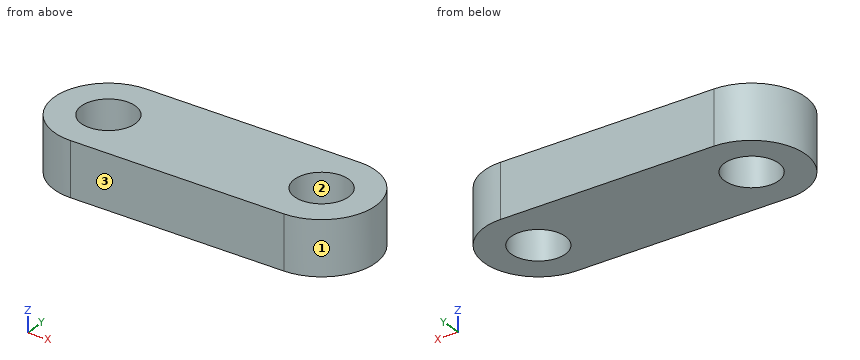
```python
from build123d import *

# Parameters (mm, degrees)
BASE_EXTRUDE_DEPTH              = 3.175
F_1_4_0_250000_DIAMETER_HOLE1_D = 6.35


with BuildPart() as part:
    # profile → Base-Extrude (new body, symmetric)
    with BuildSketch(Plane.XY):
        with BuildLine():
            Line((-25.4, 6.35), (0, 6.35))
            ThreePointArc((0, 6.35), (6.35, 0), (0, -6.35))
            Line((0, -6.35), (-25.4, -6.35))
            ThreePointArc((-25.4, -6.35), (-31.75, 0), (-25.4, 6.35))
        make_face()
    extrude(amount=BASE_EXTRUDE_DEPTH, both=True)

    # 1/4 (0.250000) Diameter Hole1 (through all)
    with Locations(Plane.XY.offset(3.175)):
        with Locations((-25.4, 0), (0, 0)):
            Hole(F_1_4_0_250000_DIAMETER_HOLE1_D / 2)


solid = part.part
```
Check sheet for the modelled part. Datum: model origin and axes. Units: mm. Face numbers are marked on the shaded views. Coordinates: 2 decimals unless noted, no trailing zeros. Order: outer loops, then holes, each group sorted by start corner. A loop starts at its lowest first (then second) coordinate and runs counter-clockwise, first axis right, second up. Notation, with made-up numbers: (-17, 60) -> (40, 60) arc R7 ccw to (40, 71) -> close; hole circle Ø5 at (48.5, 65.5). An arc over 180 degrees is marked (long way). Write item = value, one per line. Start each with the question number.
1) Cross-section at B-B (z = -1.25). Enter the section's corners in (x, y) (3 decimals).
2) Go/stop test with a flat-tipped pin: P1, Ø1.5, axis at y = -4, z = 0.5, coming from the +X side. Record where the tip stops, or that it passes through.
3) Cross-section at D-D (y = -2.25). Enter the section's corners in (x, z) (3 decimals).
4) Mould release check, pull along Y, two halves, no side actions. Record for the marked faces 1, 2 and 3: +Y half, -Y half, draft (parallel to the pull), parting line (faces both ways), or undercut.
5) Material ranges on L1, parallel to X at y = -2, z = -1.5; L2, parallel to X at y = -0.25, z = 2; L3, parallel to Y at x = -28, z = 1, recorded low to high.
6) Cross-section at A-A (y = 0). Enter the section's corners in (x, z) (3 decimals), then the cut area to 3 significant figures.
7) Cross-section at C-C (x = -26). Enter the section's corners in (y, z) (3 decimals).
Ans:
q1.outline = (-25.4, -6.35) -> (0, -6.35) arc R6.35 ccw to (0, 6.35) -> (-25.4, 6.35) arc R6.35 ccw to start; hole circle Ø6.35 at (-25.4, 0); hole circle Ø6.35 at (0, 0)
q2.P1 = 5.46
q3.outline = (-31.338, -3.175) -> (-27.64, -3.175) -> (-27.64, 3.175) -> (-31.338, 3.175) -> close; (-23.16, -3.175) -> (-2.24, -3.175) -> (-2.24, 3.175) -> (-23.16, 3.175) -> close; (2.24, -3.175) -> (5.938, -3.175) -> (5.938, 3.175) -> (2.24, 3.175) -> close
q4.face_1 = parting line
q4.face_2 = undercut
q4.face_3 = -Y half
q5.L1 = -31.43 to -27.87, -22.93 to -2.47, 2.47 to 6.03
q5.L2 = -31.75 to -28.57, -22.23 to -3.17, 3.17 to 6.35
q5.L3 = -5.79 to -1.82, 1.82 to 5.79
q6.outline = (-31.75, -3.175) -> (-28.575, -3.175) -> (-28.575, 3.175) -> (-31.75, 3.175) -> close; (-22.225, -3.175) -> (-3.175, -3.175) -> (-3.175, 3.175) -> (-22.225, 3.175) -> close; (3.175, -3.175) -> (6.35, -3.175) -> (6.35, 3.175) -> (3.175, 3.175) -> close
q6.area = 161 mm²
q7.outline = (-6.322, -3.175) -> (-3.118, -3.175) -> (-3.118, 3.175) -> (-6.322, 3.175) -> close; (3.118, -3.175) -> (6.322, -3.175) -> (6.322, 3.175) -> (3.118, 3.175) -> close
